For this review, take the finished solid that the model builds, in its own axes (mm). Face numbers are marked on the shaded views. A direction names the side the tool comes from. Coordinates: 2 decimals unless noted, no trailing zeros. Loops run counter-clockwise (first coordinate to the right, second up) from the corner with the lowest first, then second, coordinate; pieces in that order, holes last. Notation, with made-up numbers: (61, 59.5) -> (66, 59.5) arc R22 ccw to (66, 98.5) -> close; hole circle Ø3 at (20, 47.5). An arc over 180 degrees is marked (long way). Answer in a Markdown table with one row per item.
from build123d import *

# Parameters (mm, degrees)
F1_DEPTH = 25
F2_R     = 5


with BuildPart() as f1:
    # F0 (on Front) → F1 (new body)
    with BuildSketch(Plane.XZ):
        with BuildLine():
            Line((-26.664281, 4), (-26.664281, 0))
            Line((-26.664281, 0), (43.335719, 0))
            ThreePointArc((43.335719, 0), (37.978653, 10.23556), (29.255193, 17.809602))
            Line((29.255193, 17.809602), (31.407206, 11.148608))
            Line((31.407206, 11.148608), (12.375794, 5))
            Line((12.375794, 5), (7.456908, 20.225129))
            ThreePointArc((7.456908, 20.225129), (-8.926448, 10.688342), (-26.664281, 4))
        make_face()
    extrude(amount=F1_DEPTH)

    # F2
    f2_edges = [f1.edges().sort_by_distance(p)[0] for p in [
        (-26.664281, -12.5, 4),
    ]]
    fillet(f2_edges, radius=F2_R)


solid = f1.part
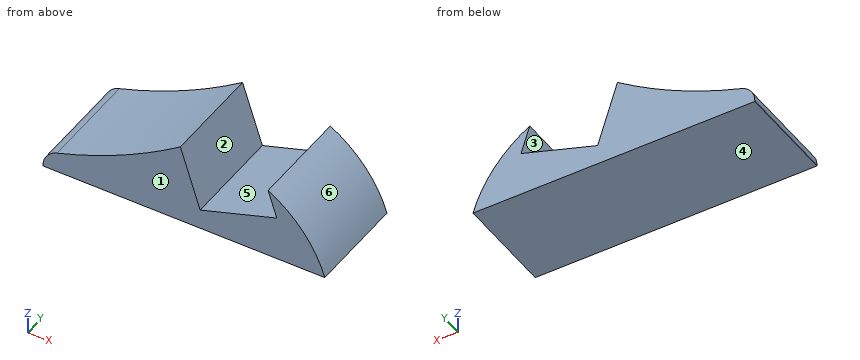
Item 1: Take a section at D-D, the plane x = -19. State the section outline as (y, z) points.
Worked answers:
| item | result |
|---|---|
| outline | (-25, 0) -> (0, 0) -> (0, 6.48) -> (-25, 6.48) -> close |
Item 2: Take a section at C-C, the plane y = -21.25. State the section outline as (x, z) points, and give its area (3 significant figures).
Worked answers:
| item | result |
|---|---|
| outline | (-26.66, 0) -> (43.34, 0) arc R31.1 ccw to (29.26, 17.81) -> (31.41, 11.15) -> (12.38, 5) -> (7.46, 20.23) arc R113.94 cw to (-23.19, 5.05) arc R5 ccw to (-26.66, 0.29) -> close |
| area | 714 mm² |
Item 3: For the marked faces 1, 2 and 3, list the 3-axis set-ups (+Z, -Z, +X, -X, +Y, -Y) from which the entire face can be reached by the end or side of a thin tool; tool diameter is ignored.
Worked answers:
| item | result |
|---|---|
| face 1 | +Z, -Z, +X, -X, -Y |
| face 2 | +Z, +Y, -Y |
| face 3 | +Y, -Y |
Item 4: Take a section at B-B, the plane z = 8.5. State the section outline as (x, y) points.
Worked answers:
| item | result |
|---|---|
| outline | (-13.82, -25) -> (11.25, -25) -> (11.25, 0) -> (-13.82, 0) -> close; (23.21, -25) -> (39.26, -25) -> (39.26, 0) -> (23.21, 0) -> close |
Item 5: Take a section at A-A, the plane x = 30. State the section outline as (y, z) points, and give its area (3 significant figures).
Worked answers:
| item | result |
|---|---|
| outline | (-25, 0) -> (0, 0) -> (0, 10.69) -> (-25, 10.69) -> close; (-25, 15.5) -> (0, 15.5) -> (0, 17.36) -> (-25, 17.36) -> close |
| area | 314 mm² |
Item 6: Insertion check: pin 1 (8 mm diameter, centred on x = -10.5, y = -17, fed in from +Z); pin 2 (5 mm diameter, centred on x = -19, z = 10.5, fed in from -Y); pin 3 (2 mm diameter, centred on x = 1.5, y = -17, fed in from +Z); pin 4 (1 mm diameter, centred on y = -6, z = 16, fed in from +X). Each pin has a flat end and moves straight along its axis. Give the tip position at first contact, or say it passes through.
Worked answers:
| item | result |
|---|---|
| pin 1 | z = 11.88 |
| pin 2 | through |
| pin 3 | z = 16.95 |
| pin 4 | x = 32.67 |
Item 7: The part is to be moulded in two halves that separate along X. For the marked faces 4, 5 and 6, say which applies: +X half, -X half, draft (parallel to the pull), parting line (faces both ways), or undercut.
Worked answers:
| item | result |
|---|---|
| face 4 | draft |
| face 5 | undercut |
| face 6 | +X half |
Item 8: For L1, parallel to Z at x = -8, y = -6; L2, parallel to X at y = -16.75, z = 12.5; L3, parallel to X at y = -4.25, z = 11.5, list the stretches that pass through material, from the lowest coordinate up.
Worked answers:
| item | result |
|---|---|
| L1 | 0 to 11.13 |
| L2 | -5.29 to 9.95, 30.97 to 36 |
| L3 | -7.25 to 10.28, 31.29 to 36.92 |
